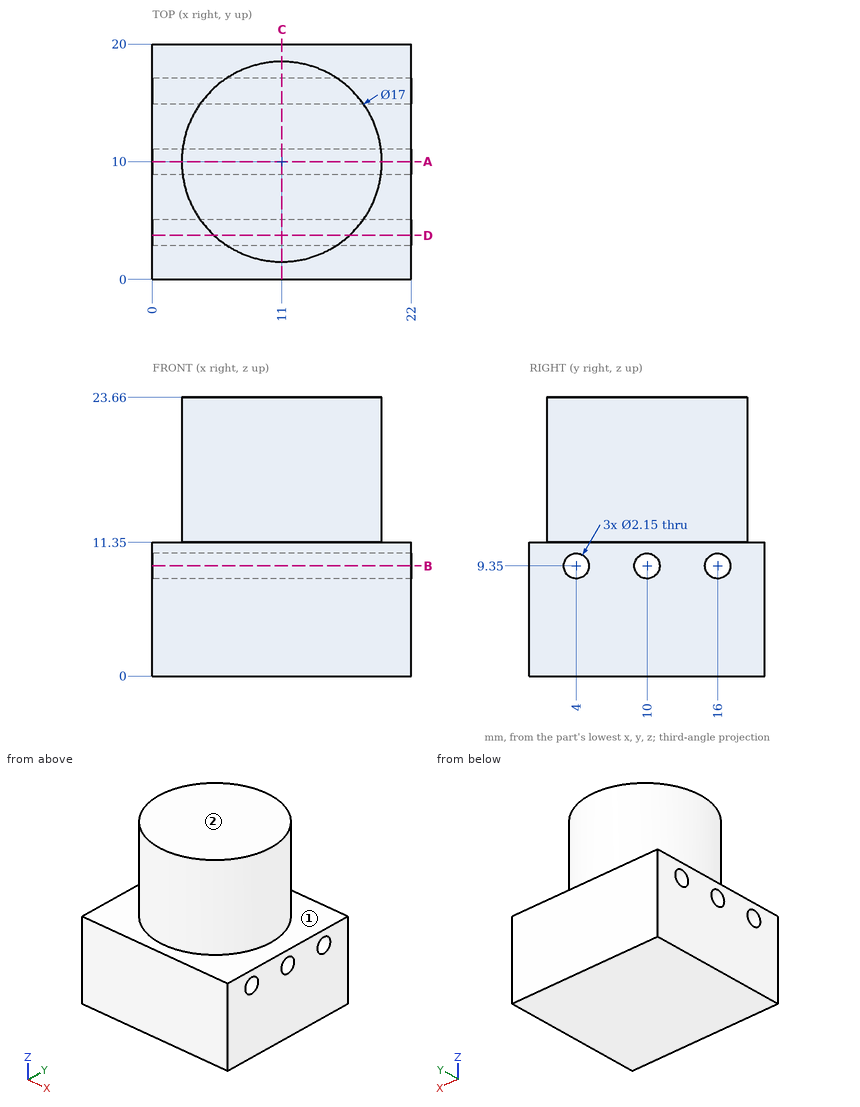
Check sheet for the drawn part. Datum: minimum x, y, z corner. Units: mm. A direction names the side the tool comes from. Give positions to 0.01 mm unless a question says otherwise; leave off trailing zeros. Loops run counter-clockwise (first coordinate to the right, second up) from the corner with the lowest first, then second, coordinate; pieces in that order, holes last. Notation, with made-up numbers: M 17,58 L 67,58 A20 cw 67,89 Z; hole C 24.5,22.25 d3. An arc over 180 degrees is marked long. Return JSON: item names as keys, results as strings.
1) Material ranges on L1, parallel to Y at x = 13.75, z = 9; L2, parallel to Z at x = 7.5, y = 4 (3 decimals); L3, parallel to Z at x = 15.75, y = 19.25, recorded low to high. Write a range as [from, to].
Findings:
{"L1": "y = [0, 2.98], [5.02, 8.98], [11.02, 14.98], [17.02, 20]", "L2": "z = [0, 8.275], [10.425, 23.66]", "L3": "z = [0, 11.35]"}
2) Section check B-B, the plane z = 9.35. Enter the section's corners in (x, y) (3 decimals).
Findings:
{"outline": "M 0,0 L 22,0 L 22,2.925 L 0,2.925 Z; M 0,5.075 L 22,5.075 L 22,8.925 L 0,8.925 Z; M 0,11.075 L 22,11.075 L 22,14.925 L 0,14.925 Z; M 0,17.075 L 22,17.075 L 22,20 L 0,20 Z"}
3) Section check D-D, the plane y = 3.75. Enter the section's corners in (x, z), and give its area (3 significant figures).
Findings:
{"outline": "M 0,0 L 22,0 L 22,8.3 L 0,8.3 Z; M 0,10.4 L 22,10.4 L 22,11.35 L 16.76,11.35 L 16.76,23.66 L 5.24,23.66 L 5.24,11.35 L 0,11.35 Z", "area": "346 mm2"}
4) Tool access check on the marked faces 1 and 2. Record the directions out of +Z, -Z, +X, -X, +Y, -Y that give a thin tool (end or side, any length) a straight path to the whole face; none if there is none.
Findings:
{"face 1": "+Z", "face 2": "+Z, +X, -X, +Y, -Y"}
5) Section check A-A, the plane y = 10. Enter the section's corners in (x, z) (3 decimals), and give its area (3 significant figures).
Findings:
{"outline": "M 0,0 L 22,0 L 22,8.275 L 0,8.275 Z; M 0,10.425 L 22,10.425 L 22,11.35 L 19.5,11.35 L 19.5,23.66 L 2.5,23.66 L 2.5,11.35 L 0,11.35 Z", "area": "412 mm2"}
6) Gauge pin test, flat ends, axial feed: P1, Ø1.5, axis at y = 15, z = 19.5, coming from the -X side; P2, Ø4, axis at x = 15, z = 21, coming from the +Y side. Record the tip position at first contact, or that the pin passes through.
Findings:
{"P1": "stops at x = 3.64", "P2": "stops at y = 18.26"}
7) Section check C-C, the plane x = 11. Enter the section's corners in (y, z) (3 decimals), and give its area (3 significant figures).
Findings:
{"outline": "M 0,0 L 20,0 L 20,11.35 L 18.5,11.35 L 18.5,23.66 L 1.5,23.66 L 1.5,11.35 L 0,11.35 Z; hole C 4,9.35 d2.15; hole C 10,9.35 d2.15; hole C 16,9.35 d2.15", "area": "425 mm2"}
